```python
from build123d import *

# Parameters (mm, degrees)
SKETCH1_R           = 2.5
BOSS_EXTRUDE1_DEPTH = 13
SKETCH2_R           = 2.609917525
SKETCH2_R_2         = 3.5
BOSS_EXTRUDE2_DEPTH = 2


with BuildPart() as part:
    # Sketch1 → Boss-Extrude1 (new body)
    with BuildSketch(Plane.XY):
        with BuildLine():
            Line((-89.768287337, 45.333507938), (-14.768287337, 45.333507938))
            ThreePointArc((-14.768287337, 45.333507938), (-6.770739373, 37.335959975), (-14.768287337, 29.338412011))
            Line((-14.768287337, 29.338412011), (-89.768287337, 29.338412011))
            ThreePointArc((-89.768287337, 29.338412011), (-97.765835301, 37.335959975), (-89.768287337, 45.333507938))
        make_face()
        with Locations((-14.768287337, 37.335959975)):
            Circle(SKETCH1_R, mode=Mode.SUBTRACT)
        with BuildLine():
            Line((-89.768287337, 40.835959975), (-77.768287337, 40.835959975))
            ThreePointArc((-77.768287337, 40.835959975), (-74.268287337, 37.335959975), (-77.768287337, 33.835959975))
            Line((-77.768287337, 33.835959975), (-89.768287337, 33.835959975))
            ThreePointArc((-89.768287337, 33.835959975), (-93.268287337, 37.335959975), (-89.768287337, 40.835959975))
        make_face(mode=Mode.SUBTRACT)
    extrude(amount=BOSS_EXTRUDE1_DEPTH)

    # Sketch2 → Boss-Extrude2 (add)
    with BuildSketch(Plane.XY.offset(13)):
        with BuildLine():
            Line((-89.768287337, 45.422284511), (-14.768287337, 45.422284511))
            ThreePointArc((-14.768287337, 45.422284511), (-6.681962801, 37.335959975), (-14.768287337, 29.249635439))
            Line((-14.768287337, 29.249635439), (-89.768287337, 29.249635439))
            ThreePointArc((-89.768287337, 29.249635439), (-97.854611873, 37.335959975), (-89.768287337, 45.422284511))
        make_face()
        with Locations((-14.768287337, 37.335959975)):
            Circle(SKETCH2_R, mode=Mode.SUBTRACT)
        with Locations((-89.768287337, 37.335959975)):
            Circle(SKETCH2_R_2, mode=Mode.SUBTRACT)
    extrude(amount=BOSS_EXTRUDE2_DEPTH)


solid = part.part
```
Model file for the job. Use its own axes, mm. A direction names the side the tool comes from. Round coordinates to 2 decimals unless told otherwise and drop trailing zeros. Loops run counter-clockwise (first coordinate to the right, second up) from the corner with the lowest first, then second, coordinate; pieces in that order, holes last. Notation, with made-up numbers: M -19.75,49.5 L 29.25,49.5 A6 cw 29.25,57.5 Z; hole C 88.5,51.25 d10. An arc over 180 degrees is marked long. Put each result on its own line as item: value. Start each with the question number.
Item 1: Cut at B-B (y = 38.5). List the corners of the cut face in (x, z), then the cut area to 3 significant figures.
Item 2: 3-axis set-ups, long thin cutter, end or side, ignore diameter. For faces 5 (the face through (-6.773, 37.512, 6.409)), 6 (the face through (-53, 45.334, 6)), 7 (the face through (-52, 37, 0)), 8 (the face through (-80, 37, 13)), 9 (the face through (-52, 29.338, 6)): which of +Z, -Z, +X, -X, +Y, -Y reach the whole face in a straight line?
Item 3: Cut at A-A (x = -82). List the corners of the cut face in (y, z), then the cut area to 3 significant figures.
Item 4: Cut at D-D (y = 31.75). List the corners of the cut face in (x, z), then the cut area to 3 significant figures.
Item 5: Mould opens along Y. For faces 1 (the face through (-12.357, 36.336, 13.986)), 2 (the face through (-52, 37, 15)), 3 (the face through (-97.764, 37.16, 6.409)), 4 (the face through (-53, 45.422, 14)) say: released by +Y, released by -Y, zero draft, split by the parting line, or undercut.
Item 6: Drill centre lines: line 1 along X through (y, z) = (39, 8.75); line 2 along Y through (x, z) = (-75.5, 8); line 3 along Y through (x, z) = (-60, 8). Where is each one in solid material? Low to high.
Item 7: Drop flat-ended pins along their axis: P1, Ø4, axis at y = 41.5, z = 7, coming from the +X side; P2, Ø4.5, axis at x = -14.77, y = 37.34, coming from the -Z side; P3, Ø1.5, axis at x = -78.5, z = 2.5, coming from the +Y side; P4, Ø1.5, axis at x = -64, z = 4, coming from the -Y side. Give the stop position or say it passes through.
Answer block:
1. outline: M -97.77,13 L -97.68,13 L -97.68,0 L -93.07,0 L -93.07,15 L -97.77,15 Z; M -86.47,13 L -74.47,13 L -74.47,0 L -16.98,0 L -16.98,13 L -17.1,13 L -17.1,15 L -86.47,15 Z; M -12.56,0 L -6.86,0 L -6.86,13 L -6.77,13 L -6.77,15 L -12.43,15 L -12.43,13 L -12.56,13 Z
1. area: 1,040 mm2
2. face 5: -Z, +X
2. face 6: -Z, +X, -X, +Y
2. face 7: -Z, +X, -X, +Y, -Y
2. face 8: -Z
2. face 9: -Z, +X, -X, -Y
3. outline: M 29.25,13 L 29.34,13 L 29.34,0 L 33.84,0 L 33.84,13 L 40.84,13 L 40.84,0 L 45.33,0 L 45.33,13 L 45.42,13 L 45.42,15 L 29.25,15 Z
3. area: 149 mm2
4. outline: M -95.62,13 L -95.49,13 L -95.49,0 L -9.04,0 L -9.04,13 L -8.92,13 L -8.92,15 L -95.62,15 Z
4. area: 1,300 mm2
5. face 1: undercut
5. face 2: zero draft
5. face 3: split by the parting line
5. face 4: released by +Y
6. line 1: -97.59 to -92.85, -74.69 to -16.63, -12.9 to -6.95
6. line 2: 29.34 to 34.67, 40 to 45.33
6. line 3: 29.34 to 45.33
7. P1: x = -7.07
7. P2: through
7. P3: y = 45.33
7. P4: y = 29.34
